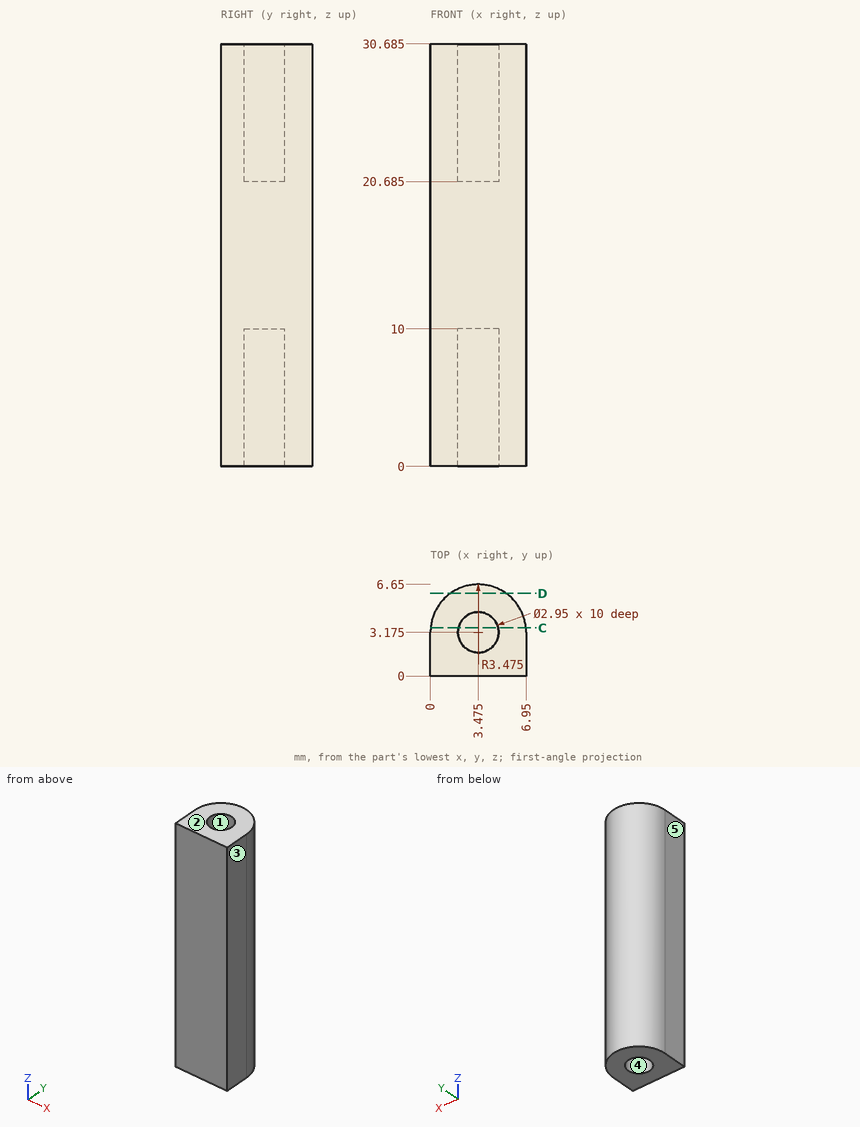
For this review, use the dimensioned drawing (mm, ordinates from the lowest corner) and the shaded views. A direction names the side the tool comes from. Give positions to 0.01 mm unless a question says otherwise; leave off trailing zeros. Loops run counter-clockwise (first coordinate to the right, second up) from the corner with the lowest first, then second, coordinate; pieces in that order, holes last.
Item 1: Take a section at D-D, the plane y = 6. State the section outline as (x, z) points (1 decimal).
Item 2: Insertion check: pin 1 (0.9 mm diameter, centred on x = 4, y = 3.5, fed in from -Z); pin 2 (1.5 mm diameter, centred on y = 5, z = 4.5, fed in from -X). Each pin has a flat end and moves straight along its axis. Give the tip position at first contact, or say it passes through.
Item 3: Draft analysis for pull direction X (two halves, no side actions). For the marked faces 1, 2 and 3, state which applies: +X half, -X half, draft (parallel to the pull), parting line (faces both ways), or undercut.
Item 4: Take a section at C-C, the plane y = 3.5. State the section outline as (x, z) points (1 decimal), and give its area (3 significant figures).
Item 5: Tool access review of the marked faces 4 and 5: name each direction out of +Z, -Z, +X, -X, +Y, -Y from which nothing blocks a thin tool from reaching the whole face with its end or side.
Item 6: For line 1 along X through (y, z) = (3.5, 21.5) (1 decimal); line 2 along Z through (x, y) = (3.5, 3.5) (1 decimal); line 3 along Y through (x, z) = (2.5, 25), list the stretches that pass through material, from the lowest coordinate up.
Calculated:
1. outline: (1.5, 0) - (5.5, 0) - (5.5, 30.7) - (1.5, 30.7) - close
2. pin 1: stops at z = 10
2. pin 2: stops at x = 0.17
3. face 1: undercut
3. face 2: draft
3. face 3: +X half
4. outline: (0, 0) - (2, 0) - (2, 10) - (4.9, 10) - (4.9, 0) - (6.9, 0) - (6.9, 30.7) - (4.9, 30.7) - (4.9, 20.7) - (2, 20.7) - (2, 30.7) - (0, 30.7) - close
4. area: 155 mm2
5. face 4: -Z
5. face 5: +Z, -Z, -X, +Y, -Y
6. line 1: x = 0 to 2, 4.9 to 6.9
6. line 2: z = 10 to 20.7
6. line 3: y = 0 to 2.07, 4.28 to 6.51
